Here's how the part is built. I have some questions about the finished solid (model axes, mm). A direction names the side the tool comes from. Give positions to 0.01 mm unless a question says otherwise; leave off trailing zeros. Order: outer loops, then holes, each group sorted by start corner. A loop starts at its lowest first (then second) coordinate and runs counter-clockwise, first axis right, second up. Notation, with made-up numbers: (87.5, 67.25) -> (137.5, 67.25) arc R31 cw to (137.5, 91.25) -> close; hole circle Ø1 at (23, 64.5). An arc over 180 degrees is marked (long way). Write each question's results on one line, items separated by ' | '. Start each with the question number.
Q1. I need wall thicknesses on line 1 along Y through (x, z) = (0, -24.25); line 2 along Z through (x, y) = (-16, 10); line 3 along Z through (x, y) = (0, 2). Which ranges of each line are inside material? Lowest first, please. Write a range as [from, to].
Q2. Imagine slicing it at A-A, the plane z = -3.5. Please give me the cut outline in (x, y).
Q3. I'm going to push flat-ended pins straight in: pin 1 (6 mm diameter, centred on x = -5.5, z = -5, fed in from -Y); pin 2 (12 mm diameter, centred on x = -12.5, y = 13, fed in from +Z); pin 3 (1 mm diameter, centred on x = 11.5, y = 2.5, fed in from +Z). Where does each tip first touch, or does it pass through?
Q4. For faces 1 (the face through (-0.17, -1.29, -25.07)), 2 (the face through (-1.08, 4.88, 3.9)), which set-ups out of +Z, -Z, +X, -X, +Y, -Y let a thin tool reach every point of the face, with its end or its side?
Q5. Imagine slicing it at B-B, the plane z = 7. State how many separate pieces and enclosed holes the cut face has, then the cut area to 3 significant figures.
Q6. Thinking about a two-plate mould opening in Y: for faces 3 (the face through (-0.17, -1.29, 4.93)), 4 (the face through (-5.48, 24.7, -10.1)), which applies, pulls with the +Y half, pulls with the -Y half, needs draft (parallel to the pull), parting line crosses it, or undercut?
```python
from build123d import *


with BuildPart() as f1:
    # F0 (on Front) → F1 (revolve)
    with BuildSketch(Plane.XZ):
        with BuildLine():
            Line((1.3, 0), (5, 0))
            Line((5, 0), (5, 7.690747))
            ThreePointArc((5, 7.690747), (13.930559, 5.375614), (22.04, 0.976557))
            ThreePointArc((22.04, 0.976557), (22.966458, -0.09252), (23.3, -1.467293))
            Line((23.3, -1.467293), (23.3, -19.010165))
            ThreePointArc((23.3, -19.010165), (22.948616, -20.419005), (21.976779, -21.497817))
            ThreePointArc((21.976779, -21.497817), (13.865739, -25.647781), (5, -27.747747))
            Line((5, -27.747747), (5, -20))
            Line((5, -20), (1.3, -20))
            Line((1.3, -20), (1.3, -30))
            ThreePointArc((1.3, -30), (13.256649, -27.968633), (24.05492, -22.447289))
            ThreePointArc((24.05492, -22.447289), (24.970651, -21.38074), (25.3, -20.014131))
            Line((25.3, -20.014131), (25.3, -0.454134))
            ThreePointArc((25.3, -0.454134), (24.985547, 0.882967), (24.108108, 1.939764))
            ThreePointArc((24.108108, 1.939764), (13.327972, 7.735387), (1.3, 10))
            Line((1.3, 10), (1.3, 0))
        make_face()
    revolve(axis=Axis((0, 0, -2.998304), (0, 0, -1)))


solid = f1.part
```
Geometry check:
1) line 1: [-21.33, -17.17], [-5, -1.3], [1.3, 5], [17.17, 21.33] | line 2: [-25.62, -23.38], [3.01, 5.29] | line 3: [-29.98, -20], [0, 9.97]
2) outline: circle Ø50.6 at (0, 0); hole circle Ø46.6 at (0, 0)
3) pin 1: y = -25.18 | pin 2: z = 8.17 | pin 3: z = 8.4
4) face 1: +Z, -Z | face 2: none
5) separate pieces: 2 | enclosed holes: 2 | area: 563 mm²
6) face 3: undercut | face 4: parting line crosses it
